from build123d import *

# Parameters (mm, degrees)
ESBO_O1_R                = 2.75
ESBO_O1_R_2              = 1.75
RESSALTO_EXTRUS_O1_DEPTH = 5
ESBO_O2_W                = 40
ESBO_O2_H                = 5.65
ESBO_O2_R                = 1.75
ESBO_O2_W_2              = 5.65
ESBO_O2_H_2              = 40
RESSALTO_EXTRUS_O2_DEPTH = 1
RESSALTO_EXTRUS_O3_DEPTH = 5
FILETE1_R                = 10


with BuildPart() as part:
    # Esboço1 → Ressalto-extrusão1 (new body)
    with BuildSketch(Plane(origin=(0, 0, 0), x_dir=(1, 0, 0), z_dir=(0, 1, 0))):
        Polygon((52.928932188, 20), (60, 20), (60, 0), (0, 0), (0, 60), (20, 60), (20, 52.928932188), (20, 20), align=None)
        with Locations(Location((10, 10, 0), (0, 0, 270))):
            Circle(ESBO_O1_R, mode=Mode.SUBTRACT)
        with Locations(Location((50, 10, 0), (0, 0, 270))):
            Circle(ESBO_O1_R_2, mode=Mode.SUBTRACT)
        with Locations(Location((10, 50, 0), (0, 0, 270))):
            Circle(ESBO_O1_R_2, mode=Mode.SUBTRACT)
    extrude(amount=RESSALTO_EXTRUS_O1_DEPTH)

    # Esboço2 → Ressalto-extrusão2 (add)
    # profile 1 of 2: a face of its own
    with BuildSketch(Plane(origin=(0, 5, 0), x_dir=(1, 0, 0), z_dir=(0, 1, 0))):
        with Locations((40, 10)):
            Rectangle(ESBO_O2_W, ESBO_O2_H)
        with Locations((50, 10)):
            Circle(ESBO_O2_R, mode=Mode.SUBTRACT)
    # profile 2 of 2: a face of its own
    with BuildSketch(Plane(origin=(0, 5, 0), x_dir=(1, 0, 0), z_dir=(0, 1, 0))):
        with Locations((10, 40)):
            Rectangle(ESBO_O2_W_2, ESBO_O2_H_2)
        with Locations((10, 50)):
            Circle(ESBO_O2_R, mode=Mode.SUBTRACT)
    extrude(amount=RESSALTO_EXTRUS_O2_DEPTH)

    # Esboço3 → Ressalto-extrusão3 (add)
    with BuildSketch(Plane.XZ):
        with BuildLine():
            Line((24.666904756, -24.666904756), (20, -20))
            Line((20, -20), (20, -46.162950904))
            Line((20, -46.162950904), (33.081475452, -33.081475452))
            Line((33.081475452, -33.081475452), (29.475230868, -29.475230868))
            ThreePointArc((29.475230868, -29.475230868), (24.666904756, -29.475230868), (24.666904756, -24.666904756))
        make_face()
        with BuildLine():
            Line((46.162950904, -20), (20, -20))
            Line((20, -20), (24.666904756, -24.666904756))
            ThreePointArc((24.666904756, -24.666904756), (28.372191482, -23.929877401), (30.471067812, -27.071067812))
            ThreePointArc((30.471067812, -27.071067812), (30.212258222, -28.372191482), (29.475230868, -29.475230868))
            Line((29.475230868, -29.475230868), (33.081475452, -33.081475452))
            Line((33.081475452, -33.081475452), (46.162950904, -20))
        make_face()
    extrude(amount=-RESSALTO_EXTRUS_O3_DEPTH)

    # Filete1
    filete1_edges = [part.edges().sort_by_distance(p)[0] for p in [
        (46.162950904, 2.5, -20),
        (20, 2.5, -46.162950904),
    ]]
    fillet(filete1_edges, radius=FILETE1_R)


solid = part.part
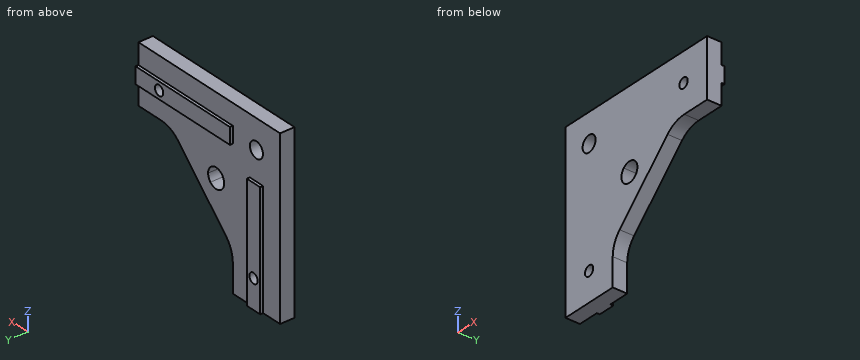
Input: part model. Units: mm. Frame: model coordinates. Coordinates: 2 decimals unless noted, no trailing zeros. Order: outer loops, then holes, each group sorted by start corner. A loop starts at its lowest first (then second) coordinate and runs counter-clockwise, first axis right, second up. Notation, with made-up numbers: M 34,6.5 L 56,6.5 A20 ccw 56,36.5 Z; hole C 40.5,-13.5 d5. An arc over 180 degrees is marked long. Write item = value, one per line. Start each with the question number.
(1) Line query: line 1 along Z through (x, y) = (8.5, 0.9); line 2 along X through (y, z) = (2.95, -10.5); line 3 along Y through (x, z) = (5, -4.5). Output: solid intervals per line, ascending. Write a range as [from, to].
(2) Section C-C on x = 32. Output: boundary loops of the cut face in (y, z) (3 decimals), and give its area (3 significant figures).
(3) Section B-B on y = 2.75. Output: boundary loops of the cut face in (x, z), and give its area (3 significant figures).
(4) First-contact query: P1, Ø0.5, axis at x = 30.5, y = 5.5, coming from the -Z side (3 decimals); P2, Ø0.8, axis at y = 5.5, z = -30, coming from the -X side (3 decimals); P3, Ø0.5, axis at y = 5.5, z = -11, coming from the -X side. Flat tips, straight axial feed; report the tip coordinate or a pass-through.
(5) Section D-D on z = -40. Output: boundary loops of the cut face in (x, y) (3 decimals), and give its area (3 significant figures).
(6) Section A-A on x = 10. Output: boundary loops of the cut face in (y, z).
Result set:
q1.line_1 = [-60, -50.9], [-49.1, -12.3], [-7.7, 0]
q1.line_2 = [0, 7.3], [12.7, 48.32], [51.68, 60]
q1.line_3 = [0, 5]
q2.outline = M 0,-34.163 L 5,-34.163 L 5,-12.825 L 6,-12.825 L 6,-7.175 L 5,-7.175 L 5,0 L 0,0 Z
q2.area = 176 mm²
q3.outline = M 0,-60 L 20,-60 L 20,-50.31 A10 cw 22.93,-43.23 L 43.23,-22.93 A10 cw 50.31,-20 L 60,-20 L 60,0 L 0,0 Z; hole C 10,-10 d5.5; hole C 10,-50 d3.5; hole C 27.07,-27.07 d6.8; hole C 50,-10 d3.5
q3.area = 2,270 mm²
q4.P1 = -12.825
q4.P2 = 7.175
q4.P3 = 20
q5.outline = M 0,0 L 26.163,0 L 26.163,5 L 12.825,5 L 12.825,6 L 7.175,6 L 7.175,5 L 0,5 Z
q5.area = 136 mm²
q6.outline = M 0,-60 L 6,-60 L 6,-51.75 L 0,-51.75 Z; M 0,-48.25 L 6,-48.25 L 6,-20 L 5,-20 L 5,-12.75 L 0,-12.75 Z; M 0,-7.25 L 5,-7.25 L 5,0 L 0,0 Z
